Drawing for the job (mm, zero at the part's lowest x, y, z). Coordinates: 2 decimals unless noted, no trailing zeros. Loops run counter-clockwise (first coordinate to the right, second up) from the corner with the lowest first, then second, coordinate; pieces in that order, holes last. Notation, with made-up numbers: (-27.75, 40) - (15.25, 40) arc R19 ccw to (15.25, 76) - close; hole circle Ø6 at (48.25, 82.5). An arc over 180 degrees is marked (long way). One line per item, written item: value.
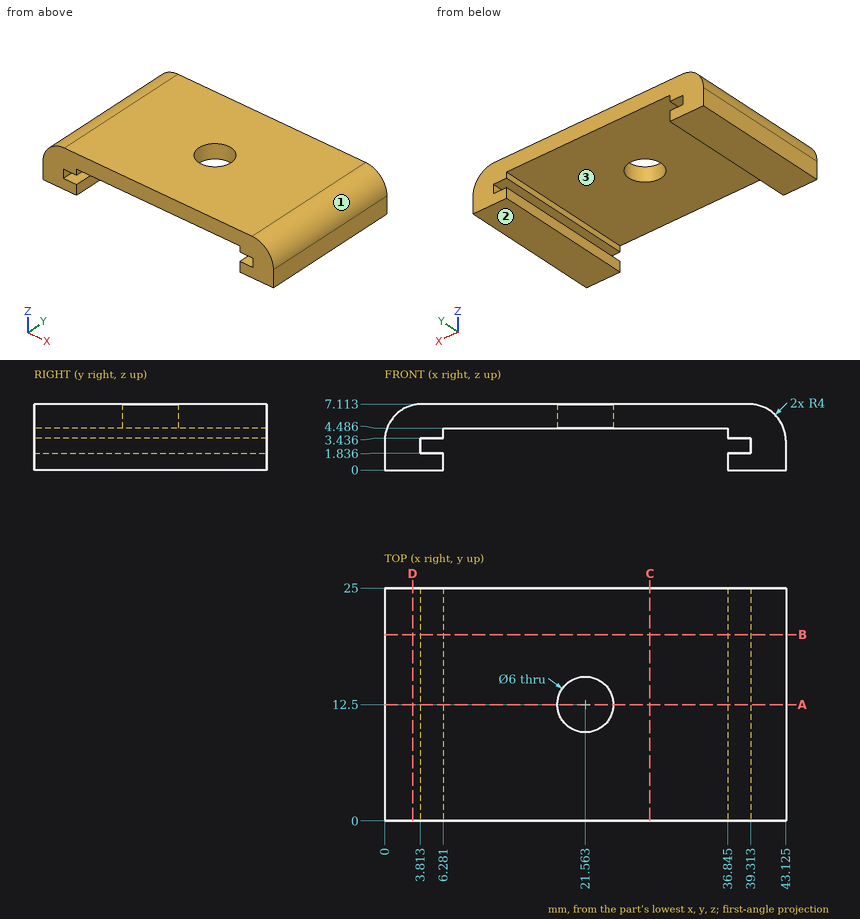
Item 1: Pull direction X, two halves, no side cores. Call the marked faces 1, 2 and 3: released by +X, released by -X, zero draft, split by the parting line, or undercut.
Check result:
face 1: released by +X
face 2: zero draft
face 3: undercut
Item 2: Cut at B-B, the plane y = 20. Write the cut outline in (x, z) (1 decimal), then the cut area to 3 significant figures.
Check result:
outline: (0, 0) - (6.3, 0) - (6.3, 1.8) - (3.8, 1.8) - (3.8, 3.4) - (6.3, 3.4) - (6.3, 4.5) - (36.8, 4.5) - (36.8, 3.4) - (39.3, 3.4) - (39.3, 1.8) - (36.8, 1.8) - (36.8, 0) - (43.1, 0) - (43.1, 3.1) arc R4 ccw to (39.1, 7.1) - (4, 7.1) arc R4 ccw to (0, 3.1) - close
area: 155 mm^2
Item 3: Drop a flat-ended pin along its axis: P1, Ø12, axis at x = 30.5, y = 14.5, coming from the -Z side. Give the stop position or say it passes through.
Check result:
P1: stops at z = 4.49
Item 4: Probe probe 1 along X at (y, z) = (12.5, 2.5) (1 decimal); probe 2 along X at (y, z) = (9, 1.75) (1 decimal); probe 3 along Z at (x, y) = (38, 14.5). List the from-to ranges inside material, lowest first. Write a range as from..to.
Check result:
probe 1: x = 0..3.8, 39.3..43.1
probe 2: x = 0..6.3, 36.8..43.1
probe 3: z = 0..1.84, 3.44..7.11
Item 5: Cut at A-A, the plane y = 12.5. Write the cut outline in (x, z) (1 decimal), then the cut area to 3 significant figures.
Check result:
outline: (0, 0) - (6.3, 0) - (6.3, 1.8) - (3.8, 1.8) - (3.8, 3.4) - (6.3, 3.4) - (6.3, 4.5) - (18.6, 4.5) - (18.6, 7.1) - (4, 7.1) arc R4 ccw to (0, 3.1) - close; (24.6, 4.5) - (36.8, 4.5) - (36.8, 3.4) - (39.3, 3.4) - (39.3, 1.8) - (36.8, 1.8) - (36.8, 0) - (43.1, 0) - (43.1, 3.1) arc R4 ccw to (39.1, 7.1) - (24.6, 7.1) - close
area: 139 mm^2
Item 6: Cut at C-C, the plane x = 28.5. Write the cut outline in (y, z).
Check result:
outline: (0, 4.49) - (25, 4.49) - (25, 7.11) - (0, 7.11) - close
Item 7: Cut at D-D, the plane x = 3. Write the cut outline in (y, z), then the cut area to 3 significant figures.
Check result:
outline: (0, 0) - (25, 0) - (25, 6.99) - (0, 6.99) - close
area: 175 mm^2
